Could you check a few things on this model? Use its own coordinates, in mm. A direction names the side the tool comes from. Coordinates: 2 decimals unless noted, no trailing zeros. Loops run counter-clockwise (first coordinate to the right, second up) from the corner with the lowest first, then second, coordinate; pieces in that order, holes last.
from build123d import *

# Parameters (mm, degrees)
F1_DEPTH = 7.62
F3_D     = 5.08
F3_DEPTH = 12.7
F4_D     = 5.08
F4_DEPTH = 12.7


with BuildPart() as f1:
    # F0 (on Top) → F1 (new body)
    with BuildSketch(Plane.XY):
        with BuildLine():
            Line((15.568078, 18.394932), (0, 18.394932))
            Line((0, 18.394932), (-15.568078, 18.394932))
            ThreePointArc((-15.568078, 18.394932), (-18.165729, 24.785284), (-23.540653, 29.109008))
            ThreePointArc((-23.540653, 29.109008), (-21.857535, 27.570607), (-21.234469, 25.377127))
            ThreePointArc((-21.234469, 25.377127), (-21.529728, 23.83544), (-22.373719, 22.511939))
            ThreePointArc((-22.373719, 22.511939), (-20.346426, 19.455849), (-20.576485, 15.795702))
            ThreePointArc((-20.576485, 15.795702), (-23.7418, -0.239949), (-20.576485, -16.2756))
            ThreePointArc((-20.576485, -16.2756), (-14.735157, -22.687615), (-6.146982, -23.903467))
            Line((-6.146982, -23.903467), (-6.146982, -25.422873))
            Line((-6.146982, -25.422873), (-23.984324, -25.422873))
            Line((-23.984324, -25.422873), (-23.984324, -27.962873))
            Line((-23.984324, -27.962873), (0, -27.962873))
            Line((0, -27.962873), (23.984324, -27.962873))
            Line((23.984324, -27.962873), (23.984324, -25.422873))
            Line((23.984324, -25.422873), (6.146982, -25.422873))
            Line((6.146982, -25.422873), (6.146982, -23.903467))
            ThreePointArc((6.146982, -23.903467), (14.735157, -22.687615), (20.576485, -16.2756))
            ThreePointArc((20.576485, -16.2756), (23.7418, -0.239949), (20.576485, 15.795702))
            ThreePointArc((20.576485, 15.795702), (20.346426, 19.455849), (22.373719, 22.511939))
            ThreePointArc((22.373719, 22.511939), (21.298254, 26.103916), (23.540653, 29.109008))
            ThreePointArc((23.540653, 29.109008), (18.165729, 24.785284), (15.568078, 18.394932))
        make_face()
        with BuildLine():
            Line((-15.568078, 15.716709), (0, 15.716709))
            Line((0, 15.716709), (15.568078, 15.716709))
            ThreePointArc((15.568078, 15.716709), (18.720393, 1.774382), (15.568078, -12.167946))
            ThreePointArc((15.568078, -12.167946), (12.222243, -16.213262), (7.349744, -18.16722))
            ThreePointArc((7.349744, -18.16722), (5.494258, -16.270557), (7.349744, -14.373895))
            Line((7.349744, -14.373895), (0, -14.373895))
            Line((0, -14.373895), (-7.349744, -14.373895))
            ThreePointArc((-7.349744, -14.373895), (-5.494258, -16.270557), (-7.349744, -18.16722))
            ThreePointArc((-7.349744, -18.16722), (-12.222243, -16.213262), (-15.568078, -12.167946))
            ThreePointArc((-15.568078, -12.167946), (-18.720393, 1.774382), (-15.568078, 15.716709))
        make_face(mode=Mode.SUBTRACT)
        with BuildLine():
            ThreePointArc((23.979965, 29.29807), (23.759487, 29.20545), (23.540653, 29.109008))
            ThreePointArc((23.540653, 29.109008), (21.298254, 26.103916), (22.373719, 22.511939))
            ThreePointArc((22.373719, 22.511939), (26.948726, 21.499817), (29.579608, 25.377127))
            ThreePointArc((29.579608, 25.377127), (27.800339, 28.795087), (23.979965, 29.29807))
        make_face()
        with BuildLine():
            ThreePointArc((-21.234469, 25.377127), (-21.857535, 27.570607), (-23.540653, 29.109008))
            ThreePointArc((-23.540653, 29.109008), (-23.759487, 29.20545), (-23.979965, 29.29807))
            ThreePointArc((-23.979965, 29.29807), (-29.467417, 24.416054), (-22.373719, 22.511939))
            ThreePointArc((-22.373719, 22.511939), (-21.529728, 23.83544), (-21.234469, 25.377127))
        make_face()
    extrude(amount=F1_DEPTH)

    # F3
    with Locations(Plane(origin=(0, 18.394932, 0), x_dir=(-1, 0, 0), z_dir=(0, 1, 0))):
        with Locations((7.784039, 3.81)):
            Hole(F3_D / 2, depth=F3_DEPTH)

    # F4
    with Locations(Plane(origin=(0, 18.394932, 0), x_dir=(-1, 0, 0), z_dir=(0, 1, 0))):
        with Locations((-7.784039, 3.81)):
            Hole(F4_D / 2, depth=F4_DEPTH)


solid = f1.part
1) Imagine slicing it at A-A on x = -17. List the corners of the cut face in (y, z) for me, plus the area to 3 significant figures.
2) Imagine slicing it at B-B on y = -11.5. List the corners of the cut face in (x, z) for me.
3) Will these pins go through, and if not, where does the flat tip stop? pin 1 (4 mm diameter, centred on x = 3.5, z = 3.5, fed in from +Y); pin 2 (4 mm diameter, centred on y = -5.5, z = 6, fed in from -X); pin 3 (1.3 mm diameter, centred on y = -27, z = 5, fed in from -X).
4) We'd pull the mould along X, two halves only. Please class faces 6 (the flat face through (0, -16, 7.62)), 7 (the cylindrical face through (10.2, 17, 4.6)), 8 (the cylindrical face through (-23.74, -0.01, 3.76)): released by +X, released by -X, zero draft, split by the parting line, or undercut.
5) Imagine slicing it at C-C on x = 25.5. List the corners of the cut face in (y, z) for me.
6) For faces 1 (the flat face through (23.984, -27, 4)), 2 (the flat face through (0, 18.395, 4)), 3 (the cylindrical face through (5.495, -16.312, 3.757)), 4 (the cylindrical face through (23.74, -0.47, 3.76)), 5 (the flat face through (0, -27.963, 4)), which set-ups out of +Z, -Z, +X, -X, +Y, -Y let a thin tool reach every point of the face, with its end or its side?
7) If I drill on L1, parallel to Y at x = 2.5, z = 5.5; L2, parallel to Y at x = 11, z = 1.5; L3, parallel to X at y = 22, z = 2.75, over which ranges is the centre line in solid material (lowest first)?
Solved:
1. outline: (-27.96, 0) - (-25.42, 0) - (-25.42, 7.62) - (-27.96, 7.62) - close; (-21.16, 0) - (-8.64, 0) - (-8.64, 7.62) - (-21.16, 7.62) - close; (12.19, 0) - (22.93, 0) - (22.93, 7.62) - (12.19, 7.62) - close
1. area: 197 mm2
2. outline: (-22.21, 0) - (-15.88, 0) - (-15.88, 7.62) - (-22.21, 7.62) - close; (15.88, 0) - (22.21, 0) - (22.21, 7.62) - (15.88, 7.62) - close
3. pin 1: stops at y = 18.39
3. pin 2: stops at x = -23.62
3. pin 3: stops at x = -23.98
4. face 6: zero draft
4. face 7: undercut
4. face 8: released by -X
5. outline: (21.21, 0) - (29.55, 0) - (29.55, 7.62) - (21.21, 7.62) - close
6. face 1: +Z, -Z, +X, -Y
6. face 2: +Z, -Z, +Y
6. face 3: +Z, -Z
6. face 4: +Z, -Z, +X
6. face 5: +Z, -Z, +X, -X, -Y
7. L1: y = -27.96 to -14.37, 15.72 to 18.39
7. L2: y = -27.96 to -25.42, -23.97 to -16.98, 15.72 to 18.39
7. L3: x = -27.86 to -22.96, -21.8 to -16.56, 16.56 to 21.8, 22.96 to 27.86
